The listing builds one solid part. Answer for the finished solid, in the listing's coordinates (mm). A direction names the side the tool comes from. Round coordinates to 2 decimals unless told otherwise and drop trailing zeros. Write each loop counter-clockwise with the first axis right and the second up, starting at its lowest first coordinate (ties: lowest second). Pieces come first, ordered by that corner, then holes. Notation, with made-up numbers: (4, -35) - (37, -35) arc R15 cw to (37, -25) - close; hole circle Ø7 at (-15.75, 5). An arc over 180 degrees is marked (long way). Answer as CSV lines item,"result". Start each with the question number.
Item 1: For a pull along X with two mould halves and no side action, classify faces 4 (the flat face through (0, 29, -10)), 5 (the flat face through (37, 2, 22.5)), 6 (the flat face through (-48.67, 15.21, 0.35)), 7 (the flat face through (10, 29, 0)) as pulls with the +X half, pulls with the -X half, needs draft (parallel to the pull), parting line crosses it, or undercut.
Item 2: Which of the six approach directions +Z, -Z, +X, -X, +Y, -Y give full straight-line access (tool end or side, diameter ignored) to faces 1 (the flat face through (12, 35, 0)), 2 (the flat face through (0, 29, 10)), 3 (the flat face through (1, 32.5, 21))?
Item 3: A cutting plane is placed at A-A on x = 0. Determine the outline of the cut face in (y, z).
Item 4: A cutting plane is placed at C-C on z = 19. Determine the outline of the cut face in (x, y).
Item 5: A cutting plane is placed at B-B on y = 40.5. Determine the outline of the cut face in (x, z).
Item 6: Straight lines are drawn through the part: line 1 along Z through (x, y) = (32, 3); line 2 along Y through (x, z) = (-25, -19.5); line 3 along X through (y, z) = (8.5, 21). For each, find the intervals that lie inside material, in ascending order. Write a range as [from, to].
Item 7: A cutting plane is placed at D-D on y = 10.5. Determine the outline of the cut face in (x, z), and give its area (3 significant figures).
Item 8: Flat-ended cylindrical pins translate along their axes: pin 1 (8 mm diameter, centred on x = -15.5, y = 17, fed in from -Z); pin 2 (13 mm diameter, centred on x = -34, z = -9.5, fed in from -Y); pin 3 (14 mm diameter, centred on x = 13.5, y = 41.5, fed in from -Z); pin 4 (14 mm diameter, centred on y = 26.5, z = 4, fed in from +X). Find the tip coordinate at first contact, or state that the pin passes through.
```python
from build123d import *

# Parameters (mm, degrees)
BOSS_EXTRUDE2_DEPTH     = 25
BOSS_EXTRUDE3_DEPTH     = 17
SKETCH3_W               = 20
SKETCH3_H               = 20
CUT_EXTRUDE1_DEPTH      = 16
CUT_EXTRUDE1_DEPTH_BACK = 36
CUT_EXTRUDE2_DEPTH      = 51
CUT_EXTRUDE2_DEPTH_BACK = 51


with BuildPart() as part:
    # Sketch1 → Boss-Extrude2 (new body, symmetric)
    with BuildSketch(Plane.XY):
        with BuildLine():
            Line((-50, 0), (-24.39, 0))
            ThreePointArc((-24.39, 0), (0, 24.39), (24.39, 0))
            Line((24.39, 0), (50, 0))
            Line((50, 0), (47.375340094, 30))
            Line((47.375340094, 30), (45.931964421, 32.5))
            Line((45.931964421, 32.5), (-45.931964421, 32.5))
            Line((-45.931964421, 32.5), (-47.375340094, 30))
            Line((-47.375340094, 30), (-50, 0))
        make_face()
    extrude(amount=BOSS_EXTRUDE2_DEPTH, both=True)

    # Sketch1<7> → Boss-Extrude3 (add, symmetric)
    with BuildSketch(Plane.XY):
        with BuildLine():
            Line((-37.271710383, 47.5), (-45.931964421, 32.5))
            Line((-45.931964421, 32.5), (45.931964421, 32.5))
            Line((45.931964421, 32.5), (37.271710383, 47.5))
            ThreePointArc((37.271710383, 47.5), (35.441583364, 49.330127019), (32.941583364, 50))
            Line((32.941583364, 50), (17.5, 50))
            Line((17.5, 50), (17.5, 35))
            Line((17.5, 35), (-15.917158097, 35))
            Line((-15.917158097, 35), (-15.917158097, 50))
            Line((-15.917158097, 50), (-32.941583364, 50))
            ThreePointArc((-32.941583364, 50), (-35.441583364, 49.330127019), (-37.271710383, 47.5))
        make_face()
    extrude(amount=BOSS_EXTRUDE3_DEPTH, both=True)

    # Sketch3 → Cut-Extrude1 (cut, two sides)
    with BuildSketch(Plane(origin=(0, 35, 0), x_dir=(1, 0, 0), z_dir=(0, 1, 0))) as cut_extrude1_sk:
        Rectangle(SKETCH3_W, SKETCH3_H)
    extrude(amount=CUT_EXTRUDE1_DEPTH, mode=Mode.SUBTRACT)
    extrude(cut_extrude1_sk.sketch, amount=-CUT_EXTRUDE1_DEPTH_BACK, mode=Mode.SUBTRACT)

    # Sketch5 → Cut-Extrude2 (cut, two sides)
    with BuildSketch(Plane(origin=(0, 0, 0), x_dir=(0, 0, -1), z_dir=(1, 0, 0))) as cut_extrude2_sk:
        Polygon((-176.421356237, 0), (-25, 0), (-22.5, 0), (-22.5, 5), (22.5, 5), (22.5, 0), (25, 0), (176.421356237, 0), (176.421356237, -302.842712475), (-176.421356237, -302.842712475), align=None)
    extrude(amount=CUT_EXTRUDE2_DEPTH, mode=Mode.SUBTRACT)
    extrude(cut_extrude2_sk.sketch, amount=-CUT_EXTRUDE2_DEPTH_BACK, mode=Mode.SUBTRACT)


solid = part.part
```
Geometry says:
1,face 4,"undercut"
1,face 5,"needs draft"
1,face 6,"pulls with the -X half"
1,face 7,"undercut"
2,face 1,"+Z, -Z, +Y"
2,face 2,"+Y, -Y"
2,face 3,"+Z, +X, -X, +Y"
3,outline,"(24.39, -25) - (32.5, -25) - (32.5, -17) - (35, -17) - (35, -10) - (24.39, -10) - close; (24.39, 10) - (35, 10) - (35, 17) - (32.5, 17) - (32.5, 25) - (24.39, 25) - close"
4,outline,"(-49.56, 5) - (-23.87, 5) arc R24.39 cw to (23.87, 5) - (49.56, 5) - (47.38, 30) - (45.93, 32.5) - (-45.93, 32.5) - (-47.38, 30) - close"
5,outline,"(-41.31, -17) - (-15.92, -17) - (-15.92, 17) - (-41.31, 17) - close; (17.5, -17) - (41.31, -17) - (41.31, 17) - (17.5, 17) - close"
6,line 1,"z = [-25, -22.5], [22.5, 25]"
6,line 2,"y = [5, 32.5]"
6,line 3,"x = [-49.26, -22.86], [22.86, 49.26]"
7,outline,"(-49.08, -25) - (-22.01, -25) - (-22.01, 25) - (-49.08, 25) - close; (22.01, -25) - (49.08, -25) - (49.08, 25) - (22.01, 25) - close"
7,area,"2,710 mm^2"
8,pin 1,"stops at z = -25"
8,pin 2,"stops at y = 5"
8,pin 3,"stops at z = -17"
8,pin 4,"stops at x = 48.29"
